from build123d import *

# Parameters (mm, degrees)
EXTRUDE_1_DEPTH     = 1.2
EXTRUDE_2_DEPTH     = 5.3
SKETCH_3_W          = 67.4
SKETCH_3_H          = 50.2
CUT_EXTRUDE_1_DEPTH = 68.344932994
CHAMFER_1_SIZE      = 1
SKETCH_5_R          = 1.585078886
CUT_EXTRUDE_2_DEPTH = 0.2
SKETCH_6_R          = 2.1
CUT_EXTRUDE_3_DEPTH = 3
EXTRUDE_3_DEPTH     = 0.5
EXTRUDE_4_DEPTH     = 4
SKETCH_10_W         = 4
SKETCH_10_H         = 12
CUT_EXTRUDE_4_DEPTH = 5
FILLET_1_R          = 1


with BuildPart() as part:
    # Sketch 1 → Extrude 1 (new body)
    with BuildSketch(Plane.XY):
        with BuildLine():
            Line((48.8, -33.5), (-48.8, -33.5))
            ThreePointArc((-48.8, -33.5), (-49.648528137, -33.148528137), (-50, -32.3))
            Line((-50, -32.3), (-50, 32.3))
            ThreePointArc((-50, 32.3), (-49.648528137, 33.148528137), (-48.8, 33.5))
            Line((-48.8, 33.5), (48.8, 33.5))
            ThreePointArc((48.8, 33.5), (49.648528137, 33.148528137), (50, 32.3))
            Line((50, 32.3), (50, -32.3))
            ThreePointArc((50, -32.3), (49.648528137, -33.148528137), (48.8, -33.5))
        make_face()
    extrude(amount=EXTRUDE_1_DEPTH)

    # Sketch 2 → Extrude 2 (add)
    with BuildSketch(Plane.XY):
        with BuildLine():
            Line((-48.8, -38.5), (48.8, -38.5))
            ThreePointArc((48.8, -38.5), (53.184062043, -36.684062043), (55, -32.3))
            Line((55, -32.3), (55, 32.3))
            ThreePointArc((55, 32.3), (53.184062043, 36.684062043), (48.8, 38.5))
            Line((48.8, 38.5), (-48.8, 38.5))
            ThreePointArc((-48.8, 38.5), (-53.184062043, 36.684062043), (-55, 32.3))
            Line((-55, 32.3), (-55, -32.3))
            ThreePointArc((-55, -32.3), (-53.184062043, -36.684062043), (-48.8, -38.5))
        make_face()
        with BuildLine():
            Line((50, -32.3), (50, 32.3))
            ThreePointArc((50, 32.3), (49.648528137, 33.148528137), (48.8, 33.5))
            Line((48.8, 33.5), (-48.8, 33.5))
            ThreePointArc((-48.8, 33.5), (-49.648528137, 33.148528137), (-50, 32.3))
            Line((-50, 32.3), (-50, -32.3))
            ThreePointArc((-50, -32.3), (-49.648528137, -33.148528137), (-48.8, -33.5))
            Line((-48.8, -33.5), (48.8, -33.5))
            ThreePointArc((48.8, -33.5), (49.648528137, -33.148528137), (50, -32.3))
        make_face(mode=Mode.SUBTRACT)
    extrude(amount=EXTRUDE_2_DEPTH)

    # Sketch 3 → Cut-Extrude 1 (cut, through all)
    with BuildSketch(Plane(origin=(0, 0, 0), x_dir=(-1, 0, 0), z_dir=(0, 0, -1))):
        with Locations((0.8, -0.6)):
            Rectangle(SKETCH_3_W, SKETCH_3_H)
    extrude(amount=-CUT_EXTRUDE_1_DEPTH, mode=Mode.SUBTRACT)

    # Chamfer 1
    chamfer_1_edges = [part.edges().sort_by_distance(p)[0] for p in [
        (32.9, -0.6, 0),
        (-0.8, -25.7, 0),
        (-34.5, -0.6, 0),
        (-0.8, 24.5, 0),
    ]]
    chamfer(chamfer_1_edges, length=CHAMFER_1_SIZE)

    # Sketch 5 → Cut-Extrude 2 (cut)
    with BuildSketch(Plane(origin=(0, 0, 0), x_dir=(-1, 0, 0), z_dir=(0, 0, -1))):
        with Locations((-46.577472533, 30.889007125)):
            Circle(SKETCH_5_R)
    extrude(amount=-CUT_EXTRUDE_2_DEPTH, mode=Mode.SUBTRACT)

    # Sketch 6 → Cut-Extrude 3 (cut)
    with BuildSketch(Plane.XY.offset(5.3)):
        with Locations((-50, -33.5)):
            Circle(SKETCH_6_R)
        with Locations((50, -33.5)):
            Circle(SKETCH_6_R)
        with Locations((50, 33.5)):
            Circle(SKETCH_6_R)
        with Locations((-50, 33.5)):
            Circle(SKETCH_6_R)
    extrude(amount=-CUT_EXTRUDE_3_DEPTH, mode=Mode.SUBTRACT)

    # Sketch 8 → Extrude 3 (add)
    with BuildSketch(Plane.XY.offset(5.3)):
        with BuildLine():
            Line((-50, -31.4), (-50, -32.4))
            ThreePointArc((-50, -32.4), (-50.777817459, -34.277817459), (-48.9, -33.5))
            Line((-48.9, -33.5), (-47.9, -33.5))
            ThreePointArc((-47.9, -33.5), (-51.48492424, -34.98492424), (-50, -31.4))
        make_face()
        with BuildLine():
            Line((47.9, -33.5), (48.9, -33.5))
            ThreePointArc((48.9, -33.5), (50.777817459, -34.277817459), (50, -32.4))
            Line((50, -32.4), (50, -31.4))
            ThreePointArc((50, -31.4), (51.48492424, -34.98492424), (47.9, -33.5))
        make_face()
        with BuildLine():
            Line((-47.9, 33.5), (-48.9, 33.5))
            ThreePointArc((-48.9, 33.5), (-50.777817459, 34.277817459), (-50, 32.4))
            Line((-50, 32.4), (-50, 31.4))
            ThreePointArc((-50, 31.4), (-51.48492424, 34.98492424), (-47.9, 33.5))
        make_face()
        with BuildLine():
            Line((50, 31.4), (50, 32.4))
            ThreePointArc((50, 32.4), (50.777817459, 34.277817459), (48.9, 33.5))
            Line((48.9, 33.5), (47.9, 33.5))
            ThreePointArc((47.9, 33.5), (51.48492424, 34.98492424), (50, 31.4))
        make_face()
    extrude(amount=-EXTRUDE_3_DEPTH)

    # Sketch 9 → Extrude 4 (add)
    with BuildSketch(Plane.XY.offset(5.3)):
        with BuildLine():
            Line((-55, 32.3), (-55, -32.3))
            ThreePointArc((-55, -32.3), (-53.184062043, -36.684062043), (-48.8, -38.5))
            Line((-48.8, -38.5), (48.8, -38.5))
            ThreePointArc((48.8, -38.5), (53.184062043, -36.684062043), (55, -32.3))
            Line((55, -32.3), (55, 32.3))
            ThreePointArc((55, 32.3), (53.184062043, 36.684062043), (48.8, 38.5))
            Line((48.8, 38.5), (-48.8, 38.5))
            ThreePointArc((-48.8, 38.5), (-53.184062043, 36.684062043), (-55, 32.3))
        make_face()
        with BuildLine():
            Line((-54, 32.3), (-54, -32.3))
            ThreePointArc((-54, -32.3), (-52.476955262, -35.976955262), (-48.8, -37.5))
            Line((-48.8, -37.5), (48.8, -37.5))
            ThreePointArc((48.8, -37.5), (52.476955262, -35.976955262), (54, -32.3))
            Line((54, -32.3), (54, 32.3))
            ThreePointArc((54, 32.3), (52.476955262, 35.976955262), (48.8, 37.5))
            Line((48.8, 37.5), (-48.8, 37.5))
            ThreePointArc((-48.8, 37.5), (-52.476955262, 35.976955262), (-54, 32.3))
        make_face(mode=Mode.SUBTRACT)
    extrude(amount=EXTRUDE_4_DEPTH)

    # Sketch 10 → Cut-Extrude 4 (cut, symmetric)
    with BuildSketch(Plane.ZY.offset(55)):
        with Locations((7.3, 26)):
            Rectangle(SKETCH_10_W, SKETCH_10_H)
    extrude(amount=CUT_EXTRUDE_4_DEPTH, both=True, mode=Mode.SUBTRACT)

    # Fillet 1
    fillet_1_edges = [part.edges().sort_by_distance(p)[0] for p in [
        (-54.5, 32, 9.3),
        (-54.5, 20, 9.3),
        (-54.5, 20, 5.3),
        (-54.5, 32, 5.3),
    ]]
    fillet(fillet_1_edges, radius=FILLET_1_R)


solid = part.part
Geometry: final body of the model. Coordinates: model frame, mm. A direction names the side the tool comes from. Give positions to 0.01 mm unless a question says otherwise; leave off trailing zeros. Loops run counter-clockwise (first coordinate to the right, second up) from the corner with the lowest first, then second, coordinate; pieces in that order, holes last. Notation, with made-up numbers: M -24.5,20.25 L 22.5,20.25 A11 cw 22.5,28.25 Z; hole C 39.25,-6.75 d11. An arc over 180 degrees is marked long. Put each result on its own line as item: value.
1) Mould query, pull axis Z, two halves, no side actions, for faces 4 (the flat face through (-50.9, -34.4, 4.8)), 5 (the flat face through (55, 0, 5)), 6 (the flat face through (47, 31, 0.2)). Classes: released by +Z, released by -Z, zero draft, split by the parting line, or undercut.
Computed values:
face 4: undercut
face 5: zero draft
face 6: released by -Z
2) Cut plane B-B, the plane x = 6.5. Return the cut outline in (y, z), plus the area to 3 significant figures.
Computed values:
outline: M -38.5,0 L -26.7,0 L -25.7,1 L -25.7,1.2 L -33.5,1.2 L -33.5,5.3 L -37.5,5.3 L -37.5,9.3 L -38.5,9.3 Z; M 24.5,1 L 25.5,0 L 38.5,0 L 38.5,9.3 L 37.5,9.3 L 37.5,5.3 L 33.5,5.3 L 33.5,1.2 L 24.5,1.2 Z
area: 80.2 mm^2
3) Cut plane A-A, the plane y = -18.5. Return the cut outline in (x, z), plus the area to 3 significant figures.
Computed values:
outline: M -55,0 L -35.5,0 L -34.5,1 L -34.5,1.2 L -50,1.2 L -50,5.3 L -54,5.3 L -54,9.3 L -55,9.3 Z; M 32.9,1 L 33.9,0 L 55,0 L 55,9.3 L 54,9.3 L 54,5.3 L 50,5.3 L 50,1.2 L 32.9,1.2 Z
area: 99.1 mm^2
4) Reachability of faces 1 (the flat face through (51, 34.5, 4.8)), 2 (the flat face through (54, 0, 7)), 3 (the cylindrical face through (-53.14, 36.73, 4.58)) from +Z, -Z, +X, -X, +Y, -Y: full face, straight path, thin tool, end or side. Return the list, or none.
Computed values:
face 1: none
face 2: +Z
face 3: +Z, -Z, -X, +Y
5) First-contact query: P1, Ø3.5, axis at x = -50, y = -33.5, coming from the +Z side; P2, Ø2, axis at x = -50, y = 33.5, coming from the +Z side. Flat tips, straight axial feed; report the tip coordinate or a pass-through.
Computed values:
P1: stops at z = 5.3
P2: stops at z = 2.3
6) Material intervals for L1, parallel to X at y = -12.5, z = 7.5; L2, parallel to Y at x = 38, z = 3; L3, parallel to Y at x = -27, z = 5.75, sorted ascending. Write a range as from..to.
Computed values:
L1: x = -55..-54, 54..55
L2: y = -38.5..-33.5, 33.5..38.5
L3: y = -38.5..-37.5, 37.5..38.5
